Geometry check sheet. Reference: the model listing, model coordinates, mm. A direction names the side the tool comes from. Give positions to 0.01 mm unless a question says otherwise; leave off trailing zeros. Order: outer loops, then holes, each group sorted by start corner. A loop starts at its lowest first (then second) coordinate and runs counter-clockwise, first axis right, second up.
```python
from build123d import *

# Parameters (mm, degrees)
F0_W     = 40
F0_H     = 40
F0_R     = 10
F1_DEPTH = 25
F2_DEPTH = 47
F3_SIZE  = 5


with BuildPart() as f1:
    # F0 (on Top) → F1 (new body)
    with BuildSketch(Plane.XY):
        Rectangle(F0_W, F0_H)
        Circle(F0_R, mode=Mode.SUBTRACT)
    extrude(amount=F1_DEPTH)

    # F0 (on Top) → F2 (join)
    with BuildSketch(Plane.XY):
        Circle(F0_R)
    extrude(amount=F2_DEPTH)

    # F3
    f3_edges = [f1.edges().sort_by_distance(p)[0] for p in [
        (0, 20, 25),
        (20, 0, 25),
        (0, -20, 0),
        (20, 0, 0),
        (0, 20, 0),
        (-20, 0, 0),
        (0, -20, 25),
        (-20, 0, 25),
        (-10, 0, 47),
    ]]
    chamfer(f3_edges, length=F3_SIZE)


solid = f1.part
```
Q1. Gauge pin test, flat ends, axial feed: P1, Ø10, axis at y = 14, z = 33.5, coming from the +X side; P2, Ø1.5, axis at x = -10, z = 25.5, coming from the -Y side; P3, Ø10, axis at x = 7, z = 27.5, coming from the -Y side. Record the tip position at first contact, or that the pin passes through.
Q2. Access from +Z, -Z, +X, -X, +Y, -Y to the whole of each face (thin tool, end or side, straight path). Record for faces 1 (the face through (-2.17, -9.76, 33.38)), 2 (the face through (18, 0, 22)).
Q3. Cross-section at D-D, the plane y = -11. Record the boundary of the cut face in (x, z), and give its area (3 significant figures).
Q4. Cross-section at A-A, the plane x = 0. Record the boundary of the cut face in (y, z), and give its area (4 significant figures).
Q5. Thickness scan on L1, parallel to Z at x = -15, y = 14; L2, parallel to X at y = 0.5, z = 38.5; L3, parallel to Z at x = 18.5, y = -2. Record the ranges inside material, lowest first.
Q6. Cross-section at C-C, the plane z = 34. Record the boundary of the cut face in (x, y), and give its area (3 significant figures).
Answers follow:
1. P1: stops at x = 4.36
1. P2: stops at y = -15.25
1. P3: stops at y = -17.5
2. face 1: +Z
2. face 2: +Z, +X, +Y, -Y
3. outline: (-20, 5) - (-15, 0) - (15, 0) - (20, 5) - (20, 20) - (15, 25) - (-15, 25) - (-20, 20) - close
3. area: 950 mm2
4. outline: (-20, 5) - (-15, 0) - (15, 0) - (20, 5) - (20, 20) - (15, 25) - (10, 25) - (10, 42) - (5, 47) - (-5, 47) - (-10, 42) - (-10, 25) - (-15, 25) - (-20, 20) - close
4. area: 1,365 mm2
5. L1: z = 0 to 25
5. L2: x = -9.99 to 9.99
5. L3: z = 3.5 to 21.5
6. outline: circle Ø20 at (0, 0)
6. area: 314 mm2
